Check sheet for the modelled part. Datum: model origin and axes. Units: mm. A direction names the side the tool comes from. Coordinates: 2 decimals unless noted, no trailing zeros. Loops run counter-clockwise (first coordinate to the right, second up) from the corner with the lowest first, then second, coordinate; pieces in that order, holes last. Notation, with made-up numbers: M 37,-9 L 89,-9 A12 ccw 89,6 Z; hole C 11,78.25 d3. An arc over 180 degrees is marked long. Answer as CSV lines item,"result". Start each with the question number.
from build123d import *

# Parameters (mm, degrees)
SKETCH2_R           = 11.811
BOSS_EXTRUDE1_DEPTH = 25.4
SKETCH4_OUTSIDE_W   = 34.016
SKETCH4_OUTSIDE_H   = 34.016
SKETCH4_OUTSIDE_R   = 9.398
CUT_EXTRUDE1_DEPTH  = 3.302
FILLET1_R           = 0.508
SKETCH5_R           = 0.889
BOSS_EXTRUDE2_DEPTH = 7.874
CUT_EXTRUDE2_START  = 10.16
SKETCH8_R           = 1.684208496
SKETCH8_W           = 2.54
SKETCH8_H           = 3.302
CUT_EXTRUDE2_DEPTH  = 28.071149866
BOSS_EXTRUDE3_START = 9.398
SKETCH10_R          = 1.016
BOSS_EXTRUDE3_DEPTH = 0.508
CIRPATTERN1_COUNT   = 2


with BuildPart() as part:
    # Sketch2 → Boss-Extrude1 (new body)
    with BuildSketch(Plane(origin=(0, 0, 0), x_dir=(0, 0, -1), z_dir=(1, 0, 0))):
        Circle(SKETCH2_R)
    extrude(amount=BOSS_EXTRUDE1_DEPTH)

    # Sketch4 outside → Cut-Extrude1 (cut)
    with BuildSketch(Plane(origin=(25.4, 0, 0), x_dir=(0, 0, -1), z_dir=(1, 0, 0))):
        Rectangle(SKETCH4_OUTSIDE_W, SKETCH4_OUTSIDE_H)
        Circle(SKETCH4_OUTSIDE_R, mode=Mode.SUBTRACT)
    extrude(amount=-CUT_EXTRUDE1_DEPTH, mode=Mode.SUBTRACT)

    # Fillet1
    fillet1_edges = [part.edges().sort_by_distance(p)[0] for p in [
        (22.098, 0, 11.811),
        (25.4, 0, 9.398),
        (0, 0, 11.811),
        (22.098, 0, 9.398),
    ]]
    fillet(fillet1_edges, radius=FILLET1_R)

    # Sketch5 → Boss-Extrude2 (add)
    with BuildSketch(Plane(origin=(25.4, 0, 0), x_dir=(0, 0, -1), z_dir=(1, 0, 0))):
        Circle(SKETCH5_R)
    extrude(amount=BOSS_EXTRUDE2_DEPTH)

    # Sketch8 → Cut-Extrude2 (cut, through all)
    with BuildSketch(Plane.XY.offset(CUT_EXTRUDE2_START)):
        with Locations((2.54, 0)):
            Circle(SKETCH8_R)
        with Locations((1.27, 0)):
            Rectangle(SKETCH8_W, SKETCH8_H)
    extrude(amount=CUT_EXTRUDE2_DEPTH, mode=Mode.SUBTRACT)

    # Sketch10 → Boss-Extrude3 (add)
    with BuildSketch(Plane.XY.offset(BOSS_EXTRUDE3_START)):
        with BuildLine():
            Line((-3.556, -1.524), (0, -1.524))
            Line((0, -1.524), (0, 1.524))
            Line((0, 1.524), (-3.556, 1.524))
            ThreePointArc((-3.556, 1.524), (-5.08, 0), (-3.556, -1.524))
        make_face()
        with Locations((-3.556, 0)):
            Circle(SKETCH10_R, mode=Mode.SUBTRACT)
    boss_extrude3 = extrude(amount=BOSS_EXTRUDE3_DEPTH)

    # CirPattern1: Boss-Extrude3 ×2 about axis
    cirpattern1_axis = Axis((0, 0, 0), (1, 0, 0))
    for i in range(1, CIRPATTERN1_COUNT):
        add(boss_extrude3.rotate(cirpattern1_axis, i * 360 / CIRPATTERN1_COUNT))


solid = part.part
Item 1: Material ranges on line 1 (X direction, y = -6.75, z = -1.5); line 2 (X direction, y = 0, z = -9.6); line 3 (X direction, y = 0, z = 10.8), recorded low to high. Write a range as from..to.
Item 2: Go/stop test with flat-tipped pins: pin 1 (2.5 mm diameter, centred on x = -2, y = -0.5, fed in from -Z); pin 2 (0.9 mm diameter, centred on x = -2, y = -0.5, fed in from +Z); pin 3 (0.8 mm diameter, centred on x = 1, z = 10.5, fed in from +Y); pin 4 (1.6 mm diameter, centred on x = -3.556, y = 0, fed in from -Z). Record where each tip stops, or that it passes through.
Item 3: Sectioned sample at C-C, the plane y = 0. Give the number of separate pieces and of enclosed holes in the cut face, and give its area (3 significant figures).
Item 4: Release check for a two-part mould opening along X. For faces 4 (the face through (-2, 0, -9.906)), 5 (the face through (4.224, -0.042, 10.974)), 6 (the face through (-4.57, 0.04, 9.65)), 7 (the face through (25.4, -2, 0)) record: released by +X, released by -X, zero draft, split by the parting line, or undercut.
Item 5: Sectioned sample at B-B, the plane z = 0. Record the boundary of the cut face in (x, y), and give its area (3 significant figures).
Item 6: Sectioned sample at A-A, the plane x = -1. Record the boundary of the cut face in (y, z), and give its area (3 significant figures).
Item 7: Sectioned sample at D-D, the plane x = 17. Record the boundary of the cut face in (y, z), and give its area (3 significant figures).
Item 8: Set-up check for faces 1 (the face through (-2, 0, 9.398)), 2 (the face through (29.28, -0.87, 0.19)), 3 (the face through (1, 1.651, 11)): record each of +Z, -Z, +X, -X, +Y, -Y from which the full face is reachable in a straight line by a thin tool's end or side.
Reply:
1,line 1,"0..25.4"
1,line 2,"-5.08..-4.57, -2.54..22.2"
1,line 3,"4.22..22.1"
2,pin 1,"z = -9.91"
2,pin 2,"z = 9.91"
2,pin 3,"y = 6.12"
2,pin 4,"through"
3,separate pieces,"3"
3,enclosed holes,"0"
3,area,"594 mm²"
4,face 4,"zero draft"
4,face 5,"undercut"
4,face 6,"undercut"
4,face 7,"released by +X"
5,outline,"M 0,-11.3 A0.51 ccw 0.51,-11.81 L 21.59,-11.81 A0.51 ccw 22.1,-11.3 L 22.1,-9.91 A0.51 cw 22.61,-9.4 L 24.89,-9.4 A0.51 ccw 25.4,-8.89 L 25.4,-0.89 L 33.27,-0.89 L 33.27,0.89 L 25.4,0.89 L 25.4,8.89 A0.51 ccw 24.89,9.4 L 22.61,9.4 A0.51 cw 22.1,9.91 L 22.1,11.3 A0.51 ccw 21.59,11.81 L 0.51,11.81 A0.51 ccw 0,11.3 Z"
5,area,"598 mm²"
6,outline,"M -1.52,-9.91 L 1.52,-9.91 L 1.52,-9.4 L -1.52,-9.4 Z; M -1.52,9.4 L 1.52,9.4 L 1.52,9.91 L -1.52,9.91 Z"
6,area,"3.10 mm²"
7,outline,"C 0,0 d23.62"
7,area,"438 mm²"
8,face 1,"-X, +Y, -Y"
8,face 2,"+X"
8,face 3,"+Z, -X"
